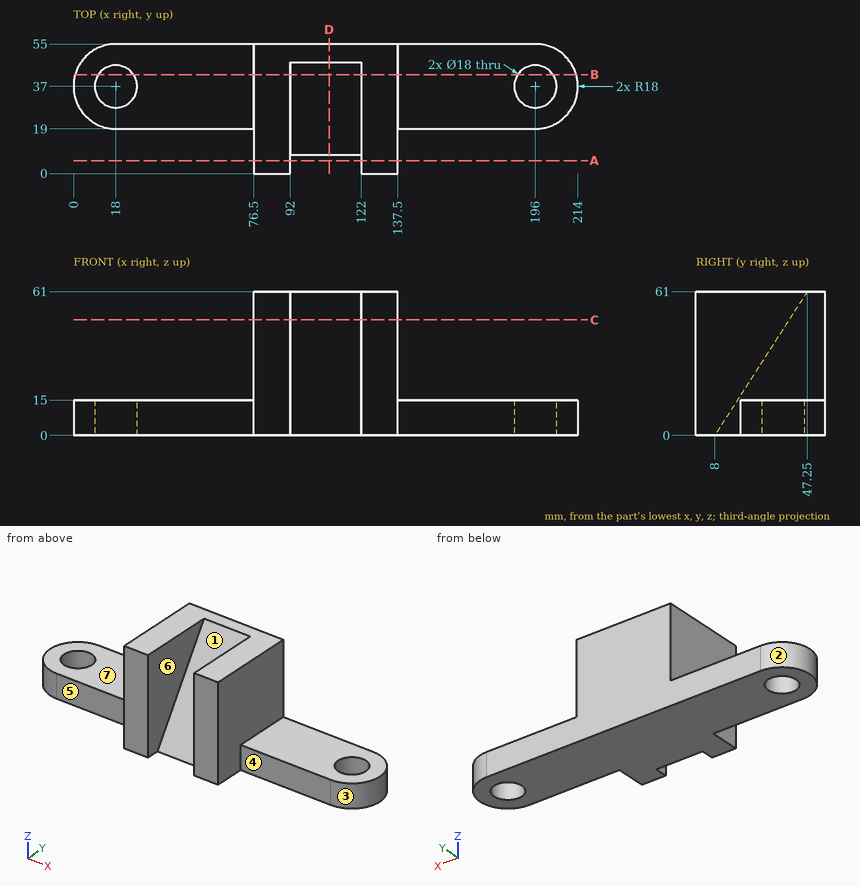
The drawing under review shows one solid part. Ordinate dimensions are in mm from its lowest x, y, z. A direction names the side the tool comes from. Round coordinates to 2 decimals unless told otherwise and drop trailing zeros. Write each loop counter-clockwise with the first axis right and the second up, starting at its lowest first coordinate (ties: lowest second). Pieces come first, ordered by that corner, then holes. Notation, with made-up numbers: (-38, -40) - (13, -40) arc R33 ccw to (13, -2) - close; hole circle Ø3 at (-23.5, -35). An arc over 180 degrees is marked (long way). Put each result on its own line as item: value.
Q1. Machinability: for the marked faces 5, 6 and 7, which of the approach directions +Z, -Z, +X, -X, +Y, -Y give a long, thin tool a straight path to every point of the face, cutting with its end or side? Answer none if there is none.
Solved:
face 5: +Z, -Z, -X, -Y
face 6: +Z, -Y
face 7: +Z, -X, +Y, -Y
Q2. Mouldability with a two-part tool opening along X and no side actions: class the marked faces 1, 2, 3 and 4 as released by +X, released by -X, zero draft, split by the parting line, or undercut.
Solved:
face 1: undercut
face 2: released by -X
face 3: released by +X
face 4: zero draft
Q3. We need section C-C (z = 49). Give the boundary of the cut face in (x, y).
Solved:
outline: (76.5, 0) - (92, 0) - (92, 39.53) - (122, 39.53) - (122, 0) - (137.5, 0) - (137.5, 55) - (76.5, 55) - close
Q4. We need section B-B (y = 42). Give the boundary of the cut face in (x, z), and give its area (3 significant figures).
Solved:
outline: (0.71, 0) - (10.52, 0) - (10.52, 15) - (0.71, 15) - close; (25.48, 0) - (188.52, 0) - (188.52, 15) - (137.5, 15) - (137.5, 61) - (122, 61) - (122, 52.84) - (92, 52.84) - (92, 61) - (76.5, 61) - (76.5, 15) - (25.48, 15) - close; (203.48, 0) - (213.29, 0) - (213.29, 15) - (203.48, 15) - close
area: 5,300 mm2
Q5. Insertion check: pin 1 Ø8 at (x, z) = (143, 20.5) entering from +Y; pin 2 Ø16.5 at (x, z) = (163.5, 7.5) entering from -Y; pin 3 Ø8 at (y, z) = (23, 11.5) entering from -X; pin 4 Ø2 at (x, y) = (160.5, 27) entering from +Z. Each pin has a flat end and moves straight along its axis. Give the tip position at first contact, or say it passes through.
Solved:
pin 1: passes through
pin 2: stops at y = 19
pin 3: stops at x = 3.03
pin 4: stops at z = 15
Q6. We need section A-A (y = 5.5). Give the boundary of the cut face in (x, z), and give its area (3 significant figures).
Solved:
outline: (76.5, 0) - (92, 0) - (92, 61) - (76.5, 61) - close; (122, 0) - (137.5, 0) - (137.5, 61) - (122, 61) - close
area: 1,890 mm2
Q7. Wall thickness on probe 1 along Y at (x, z) = (196, 3.75); probe 2 along X at (y, z) = (3, 14.5); probe 3 along Z at (x, y) = (182, 33.5): over which ranges is each line inside the solid? List them lowest first.
Solved:
probe 1: y = 19 to 28, 46 to 55
probe 2: x = 76.5 to 92, 122 to 137.5
probe 3: z = 0 to 15
Q8. We need section D-D (x = 108.5). Give the boundary of the cut face in (y, z).
Solved:
outline: (8, 0) - (55, 0) - (55, 61) - (47.25, 61) - close
